```python
from build123d import *

# Parameters (mm, degrees)
SKETCH1_W           = 25.4
SKETCH1_H           = 25.4
BOSS_EXTRUDE1_DEPTH = 5


with BuildPart() as part:
    # Sketch1 → Boss-Extrude1 (new body)
    with BuildSketch(Plane(origin=(0, 0, 0), x_dir=(1, 0, 0), z_dir=(0, 1, 0))):
        with BuildLine():
            Line((115, 160.4), (110, 160.4))
            Line((110, 160.4), (110, 176.422793918))
            ThreePointArc((110, 176.422793918), (0, 195.923209892), (-110, 176.422793918))
            Line((-110, 176.422793918), (-110, 160.4))
            Line((-110, 160.4), (-115, 160.4))
            Line((-115, 160.4), (-115, 174.545044324))
            ThreePointArc((-115, 174.545044324), (-135.614952446, 165.765554405), (-155.565, 155.565))
            ThreePointArc((-155.565, 155.565), (-165.765554405, 135.614952446), (-174.545044324, 115))
            Line((-174.545044324, 115), (-160.4, 115))
            Line((-160.4, 115), (-160.4, 110))
            Line((-160.4, 110), (-176.422793918, 110))
            ThreePointArc((-176.422793918, 110), (-195.923209892, 0), (-176.422793918, -110))
            Line((-176.422793918, -110), (-160.4, -110))
            Line((-160.4, -110), (-160.4, -115))
            Line((-160.4, -115), (-174.545044324, -115))
            ThreePointArc((-174.545044324, -115), (-165.765554405, -135.614952446), (-155.565, -155.565))
            ThreePointArc((-155.565, -155.565), (-135.614952446, -165.765554405), (-115, -174.545044324))
            Line((-115, -174.545044324), (-115, -160.4))
            Line((-115, -160.4), (-110, -160.4))
            Line((-110, -160.4), (-110, -176.422793918))
            ThreePointArc((-110, -176.422793918), (0, -195.923209892), (110, -176.422793918))
            Line((110, -176.422793918), (110, -160.4))
            Line((110, -160.4), (115, -160.4))
            Line((115, -160.4), (115, -174.545044324))
            ThreePointArc((115, -174.545044324), (135.614952446, -165.765554405), (155.565, -155.565))
            ThreePointArc((155.565, -155.565), (165.765554405, -135.614952446), (174.545044324, -115))
            Line((174.545044324, -115), (160.4, -115))
            Line((160.4, -115), (160.4, -110))
            Line((160.4, -110), (176.422793918, -110))
            ThreePointArc((176.422793918, -110), (195.923209892, 0), (176.422793918, 110))
            Line((176.422793918, 110), (160.4, 110))
            Line((160.4, 110), (160.4, 115))
            Line((160.4, 115), (174.545044324, 115))
            ThreePointArc((174.545044324, 115), (165.765554405, 135.614952446), (155.565, 155.565))
            ThreePointArc((155.565, 155.565), (135.614952446, 165.765554405), (115, 174.545044324))
            Line((115, 174.545044324), (115, 160.4))
        make_face()
        with Locations((127.7, 127.7)):
            Rectangle(SKETCH1_W, SKETCH1_H, mode=Mode.SUBTRACT)
        with Locations((-127.7, 127.7)):
            Rectangle(SKETCH1_W, SKETCH1_H, mode=Mode.SUBTRACT)
        with Locations((127.7, -127.7)):
            Rectangle(SKETCH1_W, SKETCH1_H, mode=Mode.SUBTRACT)
        with Locations((-127.7, -127.7)):
            Rectangle(SKETCH1_W, SKETCH1_H, mode=Mode.SUBTRACT)
        with BuildLine():
            ThreePointArc((-100, 100), (0, 121.301301549), (100, 100))
            ThreePointArc((100, 100), (121.301301549, 0), (100, -100))
            ThreePointArc((100, -100), (0, -121.301301549), (-100, -100))
            ThreePointArc((-100, -100), (-121.301301549, 0), (-100, 100))
        make_face(mode=Mode.SUBTRACT)
    extrude(amount=BOSS_EXTRUDE1_DEPTH)


solid = part.part
```
For this review, take the finished solid that the model builds, in its own axes (mm). A direction names the side the tool comes from. Give positions to 0.01 mm unless a question says otherwise; leave off trailing zeros. Write each loop counter-clockwise with the first axis right and the second up, starting at its lowest first coordinate (ties: lowest second). Pieces come first, ordered by that corner, then holes. Notation, with made-up numbers: M -20,9.25 L 23,9.25 A25 cw 23,44.25 Z; hole C -5,19.25 d6. An arc over 180 degrees is marked long. Answer as a JSON object with one key per item and string values. Group by question number.
Item 1: For pin 1 Ø3 at (x, y) = (133.5, 2) entering from -Z; pin 2 Ø1.5 at (x, y) = (164, 3.5) entering from +Z; pin 3 Ø2.5 at (x, y) = (125.5, 1.5) entering from -Z; pin 4 Ø3 at (x, z) = (54, -133) entering from -Y, all flat-tipped, find the tip position at first contact; note any pin that passes through.
Item 2: Consider section C-C on z = 62. Write out the cut boundary in (x, y), plus the area to 3 significant figures.
Item 3: For probe 1 along X at (y, z) = (2.25, -122.5); probe 2 along Z at (x, y) = (-163, 1.2); probe 3 along Z at (x, y) = (-168, 1.8), list the stretches that pass through material, from the lowest coordinate up. Write a range as [from, to].
Item 4: Consider section B-B on x = -82.5. Write out the cut boundary in (y, z).
Item 5: Consider section D-D on x = -169. Write out the cut boundary in (y, z), plus the area to 3 significant figures.
Item 6: Tool access review of faces 4 (the cylindrical face through (1.442, 2.465, 121.297)), 5 (the flat face through (-3, 5, -133)): name each direction out of +Z, -Z, +X, -X, +Y, -Y from which nothing blocks a thin tool from reaching the whole face with its end or side.
Item 7: Draft analysis for pull direction Z (two halves, no side actions). For faces 1 (the cylindrical face through (-1.57, 2.46, 195.92)), 2 (the cylindrical face through (-121.297, 2.465, 1.442)), 3 (the cylindrical face through (1.57, 2.46, -195.92)), state which applies: +Z half, -Z half, draft (parallel to the pull), parting line (faces both ways), or undercut.
Item 8: Consider section A-A on z = 169.5. Write out the cut boundary in (x, y).
Check result:
{
 "1": {"pin 1": "stops at z = -167.43", "pin 2": "stops at z = 140.87", "pin 3": "stops at z = -170.82", "pin 4": "stops at y = 0"},
 "2": {"outline": "M -189.86,0 L -113.34,0 L -113.34,5 L -189.86,5 Z; M 113.34,0 L 189.86,0 L 189.86,5 L 113.34,5 Z", "area": "765 mm^2"},
 "3": {"probe 1": "x = [-171.55, -140.4], [-115, 115], [140.4, 171.55]", "probe 2": "z = [-141.38, -115], [-110, 110], [115, 141.38]", "probe 3": "z = [-130.73, -115], [-110, 110], [115, 130.73]"},
 "4": {"outline": "M 0,-185.11 L 5,-185.11 L 5,-107.02 L 0,-107.02 Z; M 0,107.02 L 5,107.02 L 5,185.11 L 0,185.11 Z"},
 "5": {"outline": "M 0,-128.48 L 5,-128.48 L 5,-115 L 0,-115 Z; M 0,-110 L 5,-110 L 5,110 L 0,110 Z; M 0,115 L 5,115 L 5,128.48 L 0,128.48 Z", "area": "1,230 mm^2"},
 "6": {"face 4": "+Y, -Y", "face 5": "+Z, -Z, +X, -X, +Y"},
 "7": {"face 1": "+Z half", "face 2": "undercut", "face 3": "-Z half"},
 "8": {"outline": "M -127.33,0 L -115,0 L -115,5 L -127.33,5 Z; M -110,0 L 110,0 L 110,5 L -110,5 Z; M 115,0 L 127.33,0 L 127.33,5 L 115,5 Z"}
}
